For this review, take the finished solid that the model builds, in its own axes (mm). Face numbers are marked on the shaded views. A direction names the side the tool comes from. Coordinates: 2 decimals unless noted, no trailing zeros. Loops run counter-clockwise (first coordinate to the right, second up) from the corner with the lowest first, then second, coordinate; pieces in that order, holes last. Notation, with made-up numbers: (-15, 88.5) - (-8, 88.5) arc R24 cw to (-8, 120.5) - close; hole circle Ø9 at (15, 34.25). An arc over 180 degrees is marked (long way). One line per item, written item: value. Start each with the question number.
1. To check wall thickness, follow line 1 (X direction, y = 7.5, z = -1.75); line 2 (Z direction, x = -1, y = 2.5); line 3 (Z direction, x = -3, y = 2.25). State the ranges of each line that lie inside material, in increasing order. Write a range as from..to.
2. Take a section at D-D, the plane z = 7.25. State the section outline as (x, y) points.
3. Insertion check: pin 1 (3 mm diameter, centred on y = 11, z = 5.5, fed in from +X); pin 2 (6 mm diameter, centred on y = 1.5, z = -7, fed in from -X). Each pin has a flat end and moves straight along its axis. Give the tip position at first contact, or say it passes through.
4. Take a section at B-B, the plane z = 0. State the section outline as (x, y) points.
5. Take a section at C-C, the plane x = 0. State the section outline as (y, z) points.
6. The part is to be moulded in two halves that separate along Z. For the marked faces 1, 2 and 3, say which applies: released by +Z, released by -Z, zero draft, split by the parting line, or undercut.
7. For the marked faces 4 and 5, list the 3-axis set-ups (+Z, -Z, +X, -X, +Y, -Y) from which the entire face can be reached by the end or side of a thin tool; tool diameter is ignored.
8. Take a section at A-A, the plane y = 10.5. State the section outline as (x, z) points, and give its area (3 significant figures).
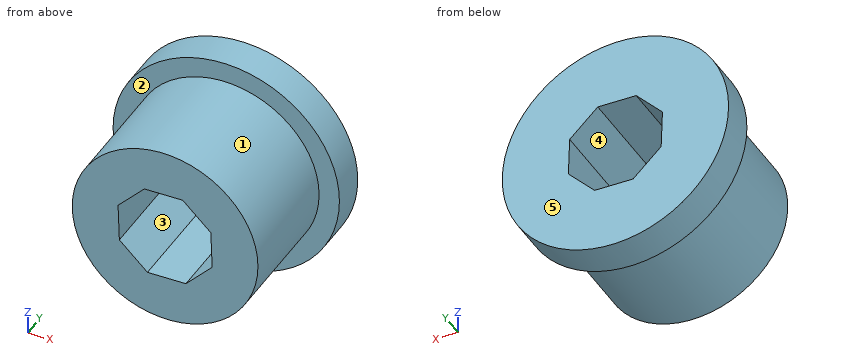
```python
from build123d import *

# Parameters (mm, degrees)
SKETCH1_R           = 8
BOSS_EXTRUDE1_DEPTH = 10
SKETCH2_R           = 9.75
BOSS_EXTRUDE2_DEPTH = 3
CUT_EXTRUDE1_DEPTH  = 14


with BuildPart() as part:
    # Sketch1 → Boss-Extrude1 (new body)
    with BuildSketch(Plane(origin=(0, 0, 0), x_dir=(1, 0, 0), z_dir=(0, 1, 0))):
        Circle(SKETCH1_R)
    extrude(amount=BOSS_EXTRUDE1_DEPTH)

    # Sketch2 → Boss-Extrude2 (add)
    with BuildSketch(Plane(origin=(0, 10, 0), x_dir=(1, 0, 0), z_dir=(0, 1, 0))):
        Circle(SKETCH2_R)
    extrude(amount=BOSS_EXTRUDE2_DEPTH)

    # Sketch3 → Cut-Extrude1 (cut, through all)
    with BuildSketch(Plane(origin=(0, 13, 0), x_dir=(1, 0, 0), z_dir=(0, 1, 0))):
        Polygon((3.941633327, -1.791282422), (4.053783603, 1.520527707), (1.791282422, 3.941633327), (-1.520527707, 4.053783603), (-3.941633327, 1.791282422), (-4.053783603, -1.520527707), (-1.791282422, -3.941633327), (1.520527707, -4.053783603), align=None)
    extrude(amount=-CUT_EXTRUDE1_DEPTH, mode=Mode.SUBTRACT)


solid = part.part
```
Solutions:
1. line 1: -7.81..-3.94, 3.84..7.81
1. line 2: -7.94..-4.04, 3.97..7.94
1. line 3: -7.42..-2.67, 2.65..7.42
2. outline: (-6.52, 10) - (-3.38, 10) - (-3.38, 0) - (3.38, 0) - (3.38, 10) - (6.52, 10) - (6.52, 13) - (-6.52, 13) - close
3. pin 1: x = 8.89
3. pin 2: x = -6.93
4. outline: (-9.75, 10) - (-8, 10) - (-8, 0) - (-4, 0) - (-4, 13) - (-9.75, 13) - close; (4, 0) - (8, 0) - (8, 10) - (9.75, 10) - (9.75, 13) - (4, 13) - close
5. outline: (0, -8) - (10, -8) - (10, -9.75) - (13, -9.75) - (13, -4) - (0, -4) - close; (0, 4) - (13, 4) - (13, 9.75) - (10, 9.75) - (10, 8) - (0, 8) - close
6. face 1: split by the parting line
6. face 2: zero draft
6. face 3: undercut
7. face 4: +Y, -Y
7. face 5: +Z, -Z, +X, -X, +Y
8. outline: circle Ø19.5 at (0, 0); hole (-4.05, 1.52) - (-3.94, -1.79) - (-1.52, -4.05) - (1.79, -3.94) - (4.05, -1.52) - (3.94, 1.79) - (1.52, 4.05) - (-1.79, 3.94) - close
8. area: 246 mm2
